Geometry check sheet. Reference: drawing and pictorial views, mm from the part's lowest x, y, z. A direction names the side the tool comes from. Round coordinates to 2 decimals unless told otherwise and drop trailing zeros. Order: outer loops, then holes, each group sorted by start corner. A loop starts at its lowest first (then second) coordinate and runs counter-clockwise, first axis right, second up.
(1) Go/stop test with flat-tipped pins: pin 1 (6 mm diameter, centred on x = 21.5, z = 56.5, fed in from +Y); pin 2 (2 mm diameter, centred on x = 7, y = 9.5, fed in from -Z); pin 3 (4 mm diameter, centred on y = 19.5, z = 50, fed in from +X). Record where each tip stops, or that it passes through.
(2) Sectioned sample at C-C (y = 12.25). Record the boundary of the cut face in (x, z), plus the area to 3 significant figures.
(3) Sectioned sample at B-B (y = 19.5). Record the boundary of the cut face in (x, z).
(4) Sectioned sample at A-A (z = 50). Record the boundary of the cut face in (x, y).
(5) Set-up check for the marked faces 1 and 2: record each of +Z, -Z, +X, -X, +Y, -Y from which the full face is reachable in a straight line by a thin tool's end or side.
(6) Release check for a two-part mould opening along X. For the marked faces 3, 4 and 5 record: +X half, -X half, draft (parallel to the pull), parting line (faces both ways), or undercut.
(7) Material ranges on line 1 along Z through (x, y) = (59, 19.25); line 2 along X through (y, z) = (10.25, 60); line 3 along Y through (x, z) = (1.55, 50), recorded low to high.
(8) Sectioned sample at D-D (x = 6.5). Record the boundary of the cut face in (y, z).
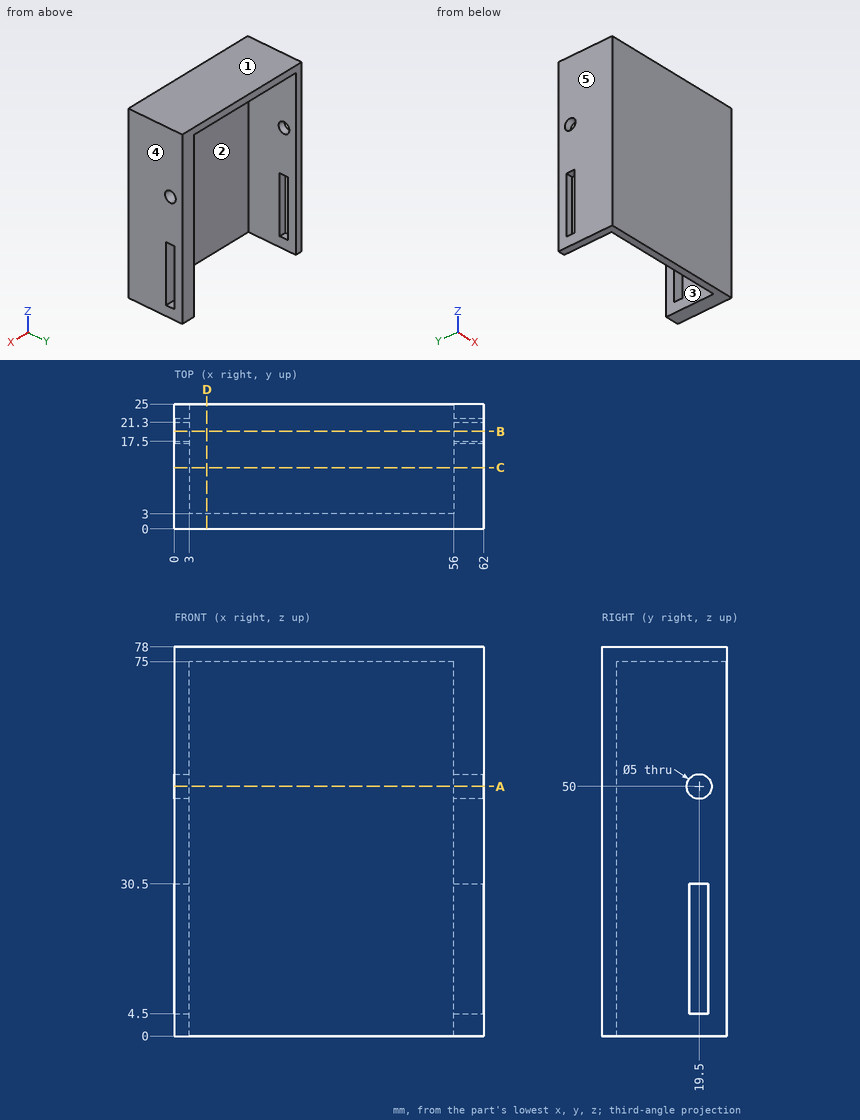
Answer below:
1. pin 1: stops at y = 3
1. pin 2: stops at z = 75
1. pin 3: passes through
2. outline: (0, 0) - (3, 0) - (3, 75) - (56, 75) - (56, 0) - (62, 0) - (62, 78) - (0, 78) - close
2. area: 861 mm2
3. outline: (0, 0) - (3, 0) - (3, 4.5) - (0, 4.5) - close; (0, 30.5) - (3, 30.5) - (3, 47.5) - (0, 47.5) - close; (0, 52.5) - (3, 52.5) - (3, 75) - (56, 75) - (56, 52.5) - (62, 52.5) - (62, 78) - (0, 78) - close; (56, 0) - (62, 0) - (62, 4.5) - (56, 4.5) - close; (56, 30.5) - (62, 30.5) - (62, 47.5) - (56, 47.5) - close
4. outline: (0, 0) - (62, 0) - (62, 17) - (56, 17) - (56, 3) - (3, 3) - (3, 17) - (0, 17) - close; (0, 22) - (3, 22) - (3, 25) - (0, 25) - close; (56, 22) - (62, 22) - (62, 25) - (56, 25) - close
5. face 1: +Z, +X, -X, +Y, -Y
5. face 2: -Z, +Y
6. face 3: undercut
6. face 4: +X half
6. face 5: -X half
7. line 1: z = 0 to 4.5, 30.5 to 47.51, 52.49 to 78
7. line 2: x = 0 to 3, 56 to 62
7. line 3: y = 0 to 17, 22 to 25
8. outline: (0, 0) - (3, 0) - (3, 75) - (25, 75) - (25, 78) - (0, 78) - close
